Build history of the part. All positions in model axes, mm. Face numbers are marked on the shaded views. A direction names the side the tool comes from. Round coordinates to 2 decimals unless told otherwise and drop trailing zeros. Order: outer loops, then holes, each group sorted by start corner. A loop starts at its lowest first (then second) coordinate and runs counter-clockwise, first axis right, second up. Notation, with made-up numbers: (-13.5, -29.5) -> (41.5, -29.5) arc R12 cw to (41.5, -9.5) -> close; hole circle Ø3 at (70.25, -24). An arc over 180 degrees is marked (long way). Write item = value, one per line.
from build123d import *

# Parameters (mm, degrees)
SKETCH3_W           = 36
SKETCH3_H           = 20
SKETCH3_R           = 2.5
BOSS_EXTRUDE2_DEPTH = 4
SKETCH4_R           = 5
BOSS_EXTRUDE3_DEPTH = 36
CHAMFER1_SIZE       = 1.5
CHAMFER1_SIZE_2     = 4.121216129
SKETCH5_W           = 10
SKETCH5_H           = 9
CUT_EXTRUDE2_DEPTH  = 45.955533586


with BuildPart() as part:
    # Sketch3 → Boss-Extrude2 (new body)
    with BuildSketch(Plane(origin=(0, 0, 0), x_dir=(0, 1, 0), z_dir=(0, 0, 1))):
        with Locations((18, 10)):
            Rectangle(SKETCH3_W, SKETCH3_H)
        with Locations(Location((8, 7.5, 0), (0, 0, 270))):
            Circle(SKETCH3_R, mode=Mode.SUBTRACT)
        with Locations(Location((28, 7.5, 0), (0, 0, 270))):
            Circle(SKETCH3_R, mode=Mode.SUBTRACT)
    extrude(amount=BOSS_EXTRUDE2_DEPTH)

    # Sketch4 → Boss-Extrude3 (add, through all)
    with BuildSketch(Plane.XZ):
        with Locations((-20, 5)):
            Circle(SKETCH4_R)
    extrude(amount=-BOSS_EXTRUDE3_DEPTH)

    # Chamfer1
    # the kernel refuses this chamfer: 4.121216129, 1.5 mm, written as the material it takes off along each edge
    with BuildSketch(Plane(origin=(-7.5, 28, 4), x_dir=(1, 0, 0), z_dir=(0, -1, 0))) as chamfer1_piece_1:
        Polygon((2.5 + CHAMFER1_SIZE, 0), (2.5, -CHAMFER1_SIZE_2), (2.5, 0), align=None)
    revolve(axis=Axis((-7.5, 28, 4), (0, 0, 1)), mode=Mode.SUBTRACT)
    with BuildSketch(Plane(origin=(-7.5, 8, 4), x_dir=(1, 0, 0), z_dir=(0, -1, 0))) as chamfer1_piece_2:
        Polygon((2.5 + CHAMFER1_SIZE, 0), (2.5, -CHAMFER1_SIZE_2), (2.5, 0), align=None)
    revolve(axis=Axis((-7.5, 8, 4), (0, 0, 1)), mode=Mode.SUBTRACT)

    # Sketch5 → Cut-Extrude2 (cut, through all)
    with BuildSketch(Plane(origin=(0, 0, 0), x_dir=(1, 0, 0), z_dir=(0, 0, -1))):
        with Locations((-20, -13.5)):
            Rectangle(SKETCH5_W, SKETCH5_H)
        with Locations((-20, -31.5)):
            Rectangle(SKETCH5_W, SKETCH5_H)
    extrude(amount=-CUT_EXTRUDE2_DEPTH, mode=Mode.SUBTRACT)


solid = part.part
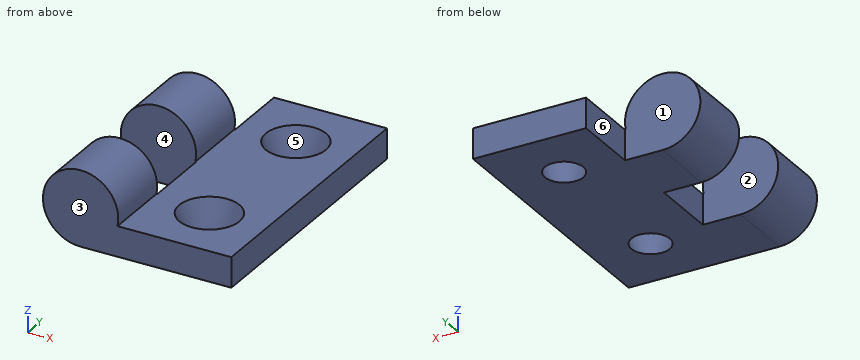
Q1. Cut at C-C, the plane x = -7.5. List the corners of the cut face in (y, z), and give its area (3 significant figures).
Check values:
outline = (0, 0) -> (5.46, 0) -> (4, 4) -> (0, 4) -> close; (10.54, 0) -> (25.46, 0) -> (24, 4) -> (12, 4) -> close; (30.54, 0) -> (36, 0) -> (36, 4) -> (32, 4) -> close
area = 91.6 mm²
Q2. Probe probe 1 along Y at (x, z) = (-22.25, 8.5); probe 2 along X at (y, z) = (12, 3); probe 3 along Z at (x, y) = (-9.25, 2). List the from-to ranges inside material, lowest first.
Check values:
probe_1 = 0 to 9, 18 to 27
probe_2 = -15 to 0
probe_3 = 0 to 4
Q3. Cut at A-A, the plane z = 5. List the corners of the cut face in (x, y).
Check values:
outline = (-25, 0) -> (-15, 0) -> (-15, 9) -> (-25, 9) -> close; (-25, 18) -> (-15, 18) -> (-15, 27) -> (-25, 27) -> close
Q4. Cut at D-D, the plane z = 3. List the corners of the cut face in (x, y).
Check values:
outline = (-24.58, 0) -> (0, 0) -> (0, 36) -> (-15, 36) -> (-15, 27) -> (-24.58, 27) -> (-24.58, 18) -> (-15, 18) -> (-15, 9) -> (-24.58, 9) -> close; hole circle Ø7.27 at (-7.5, 8); hole circle Ø7.27 at (-7.5, 28)
Q5. Mould opens along Y. For the marked faces 1, 2 and 3 say: released by +Y, released by -Y, zero draft, split by the parting line, or undercut.
Check values:
face_1 = released by +Y
face_2 = undercut
face_3 = released by -Y
Q6. Flat gauge pins, fed straight in: pin 1 (1.5 mm diameter, centred on x = -12.5, y = 12.5, fed in from +Z); pin 2 (3 mm diameter, centred on x = -20.5, z = 3.5, fed in from +Y); pin 3 (3 mm diameter, centred on y = 31, z = 3, fed in from -X). Where does each tip first touch, or does it go through?
Check values:
pin_1 = 4
pin_2 = 27
pin_3 = -15
Q7. Cut at B-B, the plane y = 8. List the corners of the cut face in (x, z), and give its area (3 significant figures).
Check values:
outline = (-20, 0) -> (-10.04, 0) -> (-11.5, 4) -> (-15.1, 4) arc R5 ccw (long way) to start; (-4.96, 0) -> (0, 0) -> (0, 4) -> (-3.5, 4) -> close
area = 118 mm²
Q8. Which spindle directions (+Z, -Z, +X, -X, +Y, -Y) get a long thin tool onto all of the face, cutting with end or side? Do the marked faces 4, 5 and 6. Say none if no direction does.
Check values:
face_4 = +Z, -Z, -X
face_5 = +Z
face_6 = +Z, -Z, -X, +Y
